Autodesk Inventor part; units mm, degrees
ref_plane "Work Plane1" through (-7.7978, 0, -7.7978) normal (0, 0, 1) x (1, 0, 0)
ref_plane "YZ Plane" through (0, 0, 0) normal (1, 0, 0) x (0, 1, 0)
ref_plane "XZ Plane" through (0, 0, 0) normal (0, 1, 0) x (-1, 0, 0)
sketch "Sketch1" plane through (0, 0, 0) normal (0, 1, 0) x (-1, 0, 0)
  line L0 (0, 0) -> (7.7978, 0)
  line L1 (7.7978, 0) -> (7.7978, -15.5956)
  line L2 (7.7978, -15.5956) -> (0, -15.5956)
  line L3 (0, -15.5956) -> (0, 0)
  dimension "d0" = 7.7978
  dimension "d1" = 15.5956
extrude "Extrusion1" add sketch "Sketch1" along normal blind 3.236
sketch "Sketch2" plane through (0, 3.236, 0) normal (0, 1, 0) x (1, 0, 0)
  line L0 (0, 0) -> (-3.8989, 0) construction
  line L1 (-3.8989, 0) -> (-3.8989, 3.8989) construction
  line L2 (-3.8989, 3.8989) -> (0, 3.8989) construction
  line L3 (0, 3.8989) -> (0, 0) construction
  circle A0 centre (-3.8989, 3.8989) radius 2.4498
  dimension "d4" = 3.8989
  dimension "d5" = 3.8989
  dimension "d6" = 4.8997
extrude "Extrusion2" add sketch "Sketch2" along normal blind 1.9837
pattern_linear "Rectangular Pattern1" count 2 spacing 7.7978 along (0, 0, -1) of "Extrusion2"
shell "Shell1" thickness 1.4732 removed faces 1 at (-2.5993, 0, -5.1985)
sketch "Sketch3" plane through (-6.3246, 1.7628, -1.4732) normal (0, -1, 0) x (1, 0, 0)
  circle A0 centre (2.4257, -2.4257) radius 2.4498 construction
  circle A1 centre (2.4257, -10.2235) radius 2.4498 construction
  circle A2 centre (2.4257, -2.4257) radius 0.9766 construction
  line L0 (2.4257, -2.4257) -> (2.4257, -10.2235) construction
  circle A3 centre (2.4257, -6.3246) radius 0.6198
  circle A4 centre (2.4257, -6.3246) radius 1.4491
  point P0 (6.3246, 1.4732)
  dimension "d13" = 1.2395
extrude "Extrusion3" add sketch "Sketch3" along normal up to surface (1.7628 mm away)
sketch "Sketch4" plane through (0, 0, 0) normal (1, 0, 0) x (0, 0, -1)
  line L0 (0, 0) -> (0, 3.236) construction
  line L1 (15.5956, 0) -> (0, 0) construction
  line L2 (0, 3.236) -> (15.5956, 0) construction
  circle A0 centre (7.7978, 1.618) radius 1.618
ref_plane "Work Plane1" through (-7.7978, 0, -7.7978) normal (0, 0, 1) x (1, 0, 0)
sketch "Sketch6" plane through (-7.7978, 0, -7.7978) normal (0, 0, 1) x (1, 0, 0)
  line L0 (7.7978, 0) -> (7.7978, 3.236)
  line L1 (7.7978, 1.618) -> (10.9982, 1.618)
  line L2 (10.9982, 1.618) -> (10.9982, 11.1506)
  dimension "d20" = 3.2004
  dimension "d21" = 9.5326
sweep "Sweep1" add profiles "Sketch4" path "Sketch6" path curves L1 L2
properties part number "1x2 short black pegged with stick thingy" material "ABS Plastic"
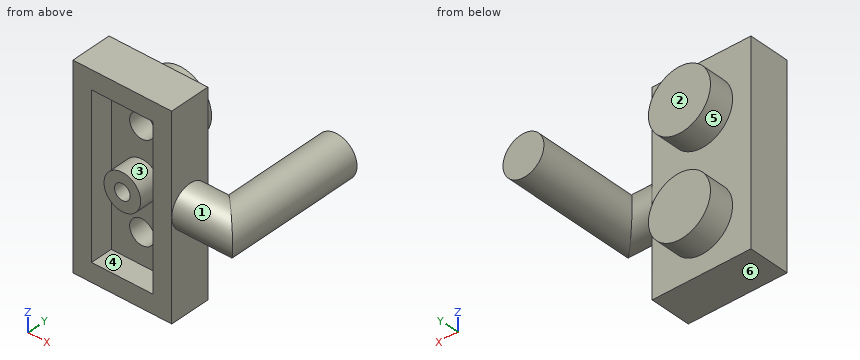
Read the model definition and answer for the solid it produces. Units are mm, in the model's axes. Face numbers are marked on the shaded views. A direction names the side the tool comes from. Give positions to 0.01 mm unless a question says otherwise; leave off trailing zeros. Loops run counter-clockwise (first coordinate to the right, second up) from the corner with the lowest first, then second, coordinate; pieces in that order, holes last.
Item 1: The part is cut by section C-C (y = 5). Write down the section's boundary in (x, z), and give its area (3 significant figures).
Item 2: Each of these flat-tipped pins is pushed along its axis until it touches: pin 1 Ø2 at (x, z) = (-3.5, -3.5) entering from -Y; pin 2 Ø5 at (x, y) = (-6, 5) entering from -Z; pin 3 Ø1.5 at (x, z) = (-5, -3.5) entering from +Y; pin 4 Ø0.9 at (y, z) = (1, -11) entering from +X. Where does it stop, or does it pass through?
Item 3: For the marked faces 4, 5 and 6, determine the directions among +Z, -Z, +X, -X, +Y, -Y from which every point of the face is accessible in a straight line to the end or side of a thin tool.
Item 4: Find the intervals of material crossed by line 1 along X through (y, z) = (1.25, -3.25); line 2 along Y through (x, z) = (-4.5, -1); line 3 along Y through (x, z) = (-3, -10.75), in increasing order.
Item 5: The part is cut by section D-D (z = -3.5). Write down the section's boundary in (x, y), and give its area (3 significant figures).
Item 6: The mould has two halves that part along Z. Classify the marked faces 1, 2 and 3: released by +Z, released by -Z, zero draft, split by the parting line, or undercut.
Item 7: The part is cut by section A-A (x = -2). Write down the section's boundary in (y, z), and give its area (3 significant figures).
Item 8: The part is cut by section B-B (z = -5.25). Write down the section's boundary in (x, y), and give its area (3 significant figures).
Taken from the geometry:
1. outline: circle Ø4.9 at (-3.9, -11.7); circle Ø4.9 at (-3.9, -3.9); circle Ø3.24 at (3.2, -7.8)
1. area: 45.9 mm2
2. pin 1: stops at y = 1.76
2. pin 2: stops at z = -15.6
2. pin 3: stops at y = 5.22
2. pin 4: stops at x = 0
3. face 4: -Y
3. face 5: +Y
3. face 6: -Z, +X, -X, +Y, -Y
4. line 1: x = -7.8 to -6.32, -1.47 to 0
4. line 2: y = 0 to 3.24
4. line 3: y = 1.76 to 5.22
5. outline: (-7.8, 0) - (-6.32, 0) - (-6.32, 1.76) - (-4.79, 1.76) - (-4.79, 3.75) - (-3.01, 3.75) - (-3.01, 1.76) - (-1.47, 1.76) - (-1.47, 0) - (0, 0) - (0, 3.24) - (-1.48, 3.24) - (-1.48, 5.22) - (-6.32, 5.22) - (-6.32, 3.24) - (-7.8, 3.24) - close
5. area: 22.7 mm2
6. face 1: split by the parting line
6. face 2: zero draft
6. face 3: undercut
7. outline: (0, -15.6) - (3.24, -15.6) - (3.24, -13.24) - (5.22, -13.24) - (5.22, -10.15) - (3.24, -10.15) - (3.24, -5.45) - (5.22, -5.45) - (5.22, -2.35) - (3.24, -2.35) - (3.24, 0) - (0, 0) - (0, -1.47) - (1.76, -1.47) - (1.76, -14.12) - (0, -14.12) - close
7. area: 40.5 mm2
8. outline: (-7.8, 0) - (-6.32, 0) - (-6.32, 1.76) - (-1.47, 1.76) - (-1.47, 0) - (0, 0) - (0, 3.24) - (-1.86, 3.24) - (-1.86, 5.22) - (-5.94, 5.22) - (-5.94, 3.24) - (-7.8, 3.24) - close
8. area: 24.8 mm2
